Build history of the part. All positions in model axes, mm. Give positions to 0.01 mm unless a question says otherwise; leave off trailing zeros. Loops run counter-clockwise (first coordinate to the right, second up) from the corner with the lowest first, then second, coordinate; pieces in that order, holes last. Notation, with made-up numbers: (-14, 20) -> (39, 20) arc R9 cw to (39, 31) -> close; hole circle Ø10 at (44, -9). An arc over 180 degrees is marked (long way). Answer as a JSON object with one key per item and string values. Group by question number.
from build123d import *

# Parameters (mm, degrees)
SKETCH1_R           = 1.55
BOSS_EXTRUDE1_DEPTH = 1.5


with BuildPart() as part:
    # Sketch1 → Boss-Extrude1 (new body)
    with BuildSketch(Plane(origin=(0, 0, 0), x_dir=(1, 0, 0), z_dir=(0, 1, 0))):
        with BuildLine():
            Line((4.973e-06, 108.599999805), (4.973e-06, 4.999999805))
            ThreePointArc((4.973e-06, 4.999999805), (1.464471067, 1.464465899), (5.000004973, -1.95e-07))
            Line((5.000004973, -1.95e-07), (365.775004973, -1.95e-07))
            ThreePointArc((365.775004973, -1.95e-07), (369.310538879, 1.464465899), (370.775004973, 4.999999805))
            Line((370.775004973, 4.999999805), (370.775004973, 108.599999805))
            ThreePointArc((370.775004973, 108.599999805), (369.310538879, 112.135533711), (365.775004973, 113.599999805))
            Line((365.775004973, 113.599999805), (5.000004973, 113.599999805))
            ThreePointArc((5.000004973, 113.599999805), (1.464471067, 112.135533711), (4.973e-06, 108.599999805))
        make_face()
        with Locations(Location((175.387504973, 109.099999805, 0), (0, 0, 270))):
            Circle(SKETCH1_R, mode=Mode.SUBTRACT)
        with Locations(Location((195.387504973, 109.099999805, 0), (0, 0, 270))):
            Circle(SKETCH1_R, mode=Mode.SUBTRACT)
        Polygon((8.000004973, 7.999999805), (8.000004973, 105.599999805), (80.387504973, 105.599999805), (83.387504973, 109.599999805), (87.387504973, 109.599999805), (90.387504973, 105.599999805), (180.387504973, 105.599999805), (183.387504973, 109.599999805), (187.387504973, 109.599999805), (190.387504973, 105.599999805), (280.387504973, 105.599999805), (283.387504973, 109.599999805), (287.387504973, 109.599999805), (290.387504973, 105.599999805), (362.775004973, 105.599999805), (362.775004973, 7.999999805), (290.387504973, 7.999999805), (287.387504973, 3.999999805), (283.387504973, 3.999999805), (280.387504973, 7.999999805), (190.387504973, 7.999999805), (187.387504973, 3.999999805), (183.387504973, 3.999999805), (180.387504973, 7.999999805), (90.387504973, 7.999999805), (87.387504973, 3.999999805), (83.387504973, 3.999999805), (80.387504973, 7.999999805), align=None, mode=Mode.SUBTRACT)
        Polygon((234.088466868, 111.349999805), (236.686543079, 111.349999805), (237.985581185, 109.099999805), (236.686543079, 106.849999805), (234.088466868, 106.849999805), (232.789428762, 109.099999805), align=None, mode=Mode.SUBTRACT)
        Polygon((334.088466868, 111.349999805), (336.686543079, 111.349999805), (337.985581185, 109.099999805), (336.686543079, 106.849999805), (334.088466868, 106.849999805), (332.789428762, 109.099999805), align=None, mode=Mode.SUBTRACT)
        Polygon((365.947436577, 110.609548716), (367.784553885, 108.772431409), (367.11212228, 106.262882498), (364.602573369, 105.590450894), (362.765456062, 107.427568201), (363.437887666, 109.937117112), align=None, mode=Mode.SUBTRACT)
        Polygon((136.686543079, 111.349999805), (134.088466868, 111.349999805), (132.789428762, 109.099999805), (134.088466868, 106.849999805), (136.686543079, 106.849999805), (137.985581185, 109.099999805), align=None, mode=Mode.SUBTRACT)
        Polygon((36.686543079, 111.349999805), (34.088466868, 111.349999805), (32.789428762, 109.099999805), (34.088466868, 106.849999805), (36.686543079, 106.849999805), (37.985581185, 109.099999805), align=None, mode=Mode.SUBTRACT)
        Polygon((4.827573369, 110.609548716), (2.990456062, 108.772431409), (3.662887666, 106.262882498), (6.172436577, 105.590450894), (8.009553885, 107.427568201), (7.33712228, 109.937117112), align=None, mode=Mode.SUBTRACT)
        Polygon((234.088466868, 2.249999805), (236.686543079, 2.249999805), (237.985581185, 4.499999805), (236.686543079, 6.749999805), (234.088466868, 6.749999805), (232.789428762, 4.499999805), align=None, mode=Mode.SUBTRACT)
        Polygon((334.088466868, 2.249999805), (336.686543079, 2.249999805), (337.985581185, 4.499999805), (336.686543079, 6.749999805), (334.088466868, 6.749999805), (332.789428762, 4.499999805), align=None, mode=Mode.SUBTRACT)
        Polygon((365.947436577, 2.990450894), (367.784553885, 4.827568201), (367.11212228, 7.337117112), (364.602573369, 8.009548716), (362.765456062, 6.172431409), (363.437887666, 3.662882498), align=None, mode=Mode.SUBTRACT)
        Polygon((136.686543079, 2.249999805), (134.088466868, 2.249999805), (132.789428762, 4.499999805), (134.088466868, 6.749999805), (136.686543079, 6.749999805), (137.985581185, 4.499999805), align=None, mode=Mode.SUBTRACT)
        Polygon((36.686543079, 2.249999805), (34.088466868, 2.249999805), (32.789428762, 4.499999805), (34.088466868, 6.749999805), (36.686543079, 6.749999805), (37.985581185, 4.499999805), align=None, mode=Mode.SUBTRACT)
        Polygon((4.827573369, 2.990450894), (2.990456062, 4.827568201), (3.662887666, 7.337117112), (6.172436577, 8.009548716), (8.009553885, 6.172431409), (7.33712228, 3.662882498), align=None, mode=Mode.SUBTRACT)
    extrude(amount=-BOSS_EXTRUDE1_DEPTH)


solid = part.part
(1) Saw through at C-C on y = -0.5. Give the number of separate pieces and of enclosed holes in the cut face, plus the area to 3 significant figures.
(2) Saw through at A-A on x = 242. List the corners of the cut face in (y, z).
(3) Probe line 1 along Z through (x, y) = (155, -0.45); line 2 along Z through (x, y) = (287, -0.1); line 3 along X through (y, z) = (-0.7, -102.5) (3 decimals). List the from-to ranges inside material, lowest first. Write a range as [from, to].
(4) Saw through at B-B on z = -21.5. List the corners of the cut face in (x, y) (3 decimals).
(5) Pin check, flat tip, straight feed: pin 1 (3 mm diameter, centred on x = 195.39, z = -109.1, fed in from -Y). Stop position of the tip, or through.
Calculated:
{
 "1": {"separate pieces": "1", "enclosed holes": "15", "area": "7,080 mm^2"},
 "2": {"outline": "(-1.5, -113.6) -> (0, -113.6) -> (0, -105.6) -> (-1.5, -105.6) -> close; (-1.5, -8) -> (0, -8) -> (0, 0) -> (-1.5, 0) -> close"},
 "3": {"line 1": "z = [-113.6, -105.6], [-8, 0]", "line 2": "z = [-113.6, -109.6], [-4, 0]", "line 3": "x = [0, 8], [362.775, 370.775]"},
 "4": {"outline": "(0, -1.5) -> (8, -1.5) -> (8, 0) -> (0, 0) -> close; (362.775, -1.5) -> (370.775, -1.5) -> (370.775, 0) -> (362.775, 0) -> close"},
 "5": {"pin 1": "passes through"}
}
